Model file for the job. Use its own axes, mm. Face numbers are marked on the shaded views. A direction names the side the tool comes from. Give positions to 0.01 mm unless a question says otherwise; leave off trailing zeros. Loops run counter-clockwise (first coordinate to the right, second up) from the corner with the lowest first, then second, coordinate; pieces in that order, holes last. Notation, with made-up numbers: (-12.5, 66.25) - (26.5, 66.25) arc R25 ccw to (26.5, 90.25) - close; hole circle Ø8 at (19, 36). An arc over 180 degrees is marked (long way). Use a Markdown table: item, result.
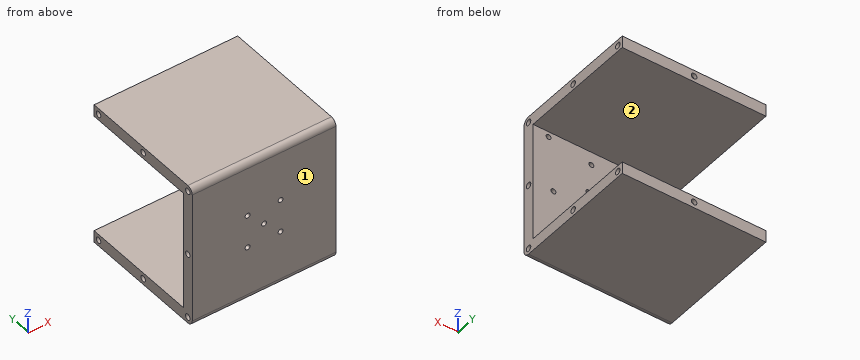
Autodesk Inventor part; units mm, degrees
ref_plane "YZ Plane" through (0, 0, 0) normal (1, 0, 0) x (0, 1, 0)
ref_plane "XZ Plane" through (0, 0, 0) normal (0, 1, 0) x (-1, 0, 0)
ref_plane "XY Plane" through (0, 0, 0) normal (0, 0, 1) x (1, 0, 0)
sketch "Sketch1" plane through (0, 0, 0) normal (0, 1, 0) x (-1, 0, 0)
  point P0 (0, 0)
sketch "Sketch2" plane through (0, 0, 0) normal (0, 1, 0) x (-1, 0, 0)
  line L0 (-76.2, 76.2) -> (76.2, 76.2)
  line L1 (76.2, 76.2) -> (76.2, -76.2)
  line L2 (76.2, -76.2) -> (-76.2, -76.2)
  line L3 (-76.2, -76.2) -> (-76.2, 76.2)
  line L4 (-76.2, 76.2) -> (76.2, -76.2) construction
  line L5 (76.2, 76.2) -> (-76.2, -76.2) construction
  point P0 (0, 0)
  dimension "d0" = 152.4
  dimension "d1" = 152.4
extrude "Extrusion1" add sketch "Sketch2" along normal blind 12.7
sketch "Sketch3" plane through (0, 12.7, 0) normal (0, 1, 0) x (1, 0, 0)
  line L0 (76.2, 76.2) -> (-76.2, 76.2)
  line L1 (76.2, -76.2) -> (76.2, 76.2)
  line L2 (-76.2, 76.2) -> (76.2, 76.2)
  line L3 (76.2, 76.2) -> (76.2, 63.5)
  line L4 (76.2, 63.5) -> (-76.2, 63.5)
  line L5 (-76.2, 63.5) -> (-76.2, 76.2)
  line L6 (-76.2, -76.2) -> (76.2, -76.2)
  line L7 (76.2, -76.2) -> (76.2, -63.5)
  line L8 (76.2, -63.5) -> (-76.2, -63.5)
  line L9 (-76.2, -63.5) -> (-76.2, -76.2)
  point P0 (0, 0)
  point P1 (76.2, -76.2)
  dimension "d4" = 12.7
  dimension "d5" = 12.7
  dimension "d15" = 152.4
extrude "Extrusion2" add sketch "Sketch3" along normal blind 127
fillet "Fillet1" radius 6.35 2 edges at (0, 0, 76.2) (0, 0, -76.2)
sketch "Sketch4" plane through (76.2, 12.7, -63.5) normal (1, 0, 0) x (0, 0, -1)
  circle A0 centre (-133.35, 120.65) radius 3.175
  circle A1 centre (-133.35, -6.35) radius 3.175
  circle A2 centre (-133.35, 57.15) radius 3.175
  circle A3 centre (6.35, 120.65) radius 3.175
  circle A4 centre (6.35, -6.35) radius 3.175
  circle A5 centre (6.35, 57.15) radius 3.175
  circle A6 centre (-63.5, -6.35) radius 3.175
  point P0 (-63.5, -12.7)
  dimension "d9" = 127
extrude "Extrusion3" cut sketch "Sketch4" against normal blind 12.7
sketch "Sketch5" plane through (-76.2, 12.7, 63.5) normal (-1, 0, 0) x (0, 0, 1)
  circle A0 centre (-133.35, 120.65) radius 3.175
  circle A1 centre (-133.35, 120.65) radius 3.175
  circle A2 centre (-133.35, 57.15) radius 3.175
  circle A3 centre (-133.35, 57.15) radius 3.175
  circle A4 centre (-133.35, -6.35) radius 3.175
  circle A5 centre (-133.35, -6.35) radius 3.175
  circle A6 centre (-63.5, -6.35) radius 3.175
  circle A7 centre (-63.5, -6.35) radius 3.175
  circle A8 centre (6.35, -6.35) radius 3.175
  circle A9 centre (6.35, -6.35) radius 3.175
  circle A10 centre (6.35, 57.15) radius 3.175
  circle A11 centre (6.35, 57.15) radius 3.175
  circle A12 centre (6.35, 120.65) radius 3.175
  circle A13 centre (6.35, 120.65) radius 3.175
  line L0 (6.35, -12.7) -> (-133.35, -12.7)
  point P0 (-63.5, -12.7)
  dimension "d20" = 69.85
sketch "Sketch6" plane through (0, 139.7, 0) normal (0, 1, 0) x (1, 0, 0)
  line L0 (76.2, 69.85) -> (-76.2, 69.85)
  circle A0 centre (0, 69.85) radius 3
  line L1 (-76.2, -69.85) -> (76.2, -69.85)
  circle A1 centre (0, -69.85) radius 3
  point P0 (0, 0)
  dimension "d16" = 6
  dimension "d17" = 6
extrude "Extrusion5" cut sketch "Sketch6" against normal blind 4
extrude "Extrusion6" cut sketch "Sketch5" against normal blind 12.7
sketch "Sketch7" plane through (0, 12.7, 0) normal (0, 1, 0) x (1, 0, 0)
  line L0 (76.2, 0) -> (63.5, 0)
  line L1 (63.5, 3.175) -> (63.5, -3.175)
  line L2 (63.5, 0) -> (57.15, 0)
  circle A0 centre (54.5465, 0) radius 2.6035
  line L3 (51.943, 0) -> (-35.687, 0)
  line L4 (-35.687, 0) -> (-35.687, 35.56)
  line L5 (-35.687, 35.56) -> (-35.687, -35.56)
  circle A1 centre (-35.687, 38.1635) radius 2.6035
  circle A2 centre (-35.687, -38.1635) radius 2.6035
  point P0 (0, 0)
  dimension "d28" = 5.207
  dimension "d29" = 5.207
  dimension "d23" = 6.35
  dimension "d24" = 5.207
  dimension "d25" = 87.63
  dimension "d26" = 35.56
  dimension "d27" = 71.12
extrude "Extrusion7" cut sketch "Sketch7" against normal blind 3.9878
sketch "Sketch8" plane through (0, 12.7, 0) normal (0, 1, 0) x (1, 0, 0)
  circle A0 centre (54.5465, 0) radius 2.6035
  line L0 (51.943, 0) -> (-76.2, 0)
  point P0 (0, 0)
sketch "Sketch9" plane through (0, 12.7, 0) normal (0, 1, 0) x (1, 0, 0)
  point P0 (0, 0)
sketch "Sketch10" plane through (0, 12.7, 0) normal (0, 1, 0) x (1, 0, 0)
  line L0 (57.15, -63.5) -> (57.15, -52.07)
  line L1 (57.15, -57.785) -> (-19.177, -57.785)
  line L2 (-76.2, -63.5) -> (76.2, -63.5)
  line L3 (13.97, -63.5) -> (13.97, -52.07)
  line L4 (11.1125, -52.07) -> (17.4625, -52.07)
  circle A0 centre (14.2875, -49.4665) radius 2.6035
  circle A1 centre (59.7535, -57.785) radius 2.6035
  line L5 (-19.177, -61.9125) -> (-19.177, -53.133)
  circle A2 centre (-21.7805, -57.785) radius 2.6035
  point P0 (0, 0)
  dimension "d32" = 11.43
  dimension "d33" = 76.327
  dimension "d36" = 5.207
  dimension "d37" = 5.207
  dimension "d38" = 5.207
extrude "Extrusion8" cut sketch "Sketch10" against normal blind 3.9878 contours A2 | A0 | A1
sketch "Sketch11" plane through (0, 0, 0) normal (0, -1, 0) x (1, 0, 0)
  line L0 (17.526, -17.526) -> (-17.526, -17.526)
  line L1 (-17.526, -17.526) -> (-17.526, 17.526)
  line L2 (-17.526, 17.526) -> (17.526, 17.526)
  line L3 (17.526, 17.526) -> (17.526, -17.526)
  line L4 (17.526, -17.526) -> (-17.526, 17.526) construction
  line L5 (-17.526, -17.526) -> (17.526, 17.526) construction
  circle A0 centre (-50.8, 55.5625) radius 2.6035
  circle A1 centre (-17.526, 17.526) radius 2.6035
  circle A2 centre (-17.526, -17.526) radius 2.6035
  circle A3 centre (17.526, -17.526) radius 2.6035
  circle A4 centre (17.526, 17.526) radius 2.6035
  point P0 (0, 0)
  dimension "d39" = 35.052
  dimension "d40" = 35.052
  dimension "d41" = 5.207
  dimension "d42" = 5.207
  dimension "d43" = 5.207
  dimension "d44" = 5.207
  dimension "d45" = 5.207
extrude "Extrusion9" cut sketch "Sketch11" along normal blind 25.4 and the other way blind 25.4 contours A2 L1 L0 | L0 L1 A2 | A3 L3 L0 | L0 L3 A3 | A1 L2 L1 | L1 L2 A1 | A4 L2 L3 | L3 L2 A4
sketch "Sketch13" plane through (0, 12.7, 0) normal (0, 1, 0) x (1, 0, 0)
  circle A0 centre (0, 0) radius 2.6035
  dimension "d54" = 5.207
extrude "Extrusion11" cut sketch "Sketch13" against normal blind 25.4
properties part number "Fuselage_Body_Piece"
(1) Slice it at C-C, the plane y = 50. Write the cut outline in (x, z), plus the area to 3 significant figures.
Computed:
| item | result |
|---|---|
| outline | (-76.2, -76.2) - (76.2, -76.2) - (76.2, -63.5) - (-76.2, -63.5) - close; (-76.2, 63.5) - (76.2, 63.5) - (76.2, 76.2) - (-76.2, 76.2) - close |
| area | 3,870 mm² |
(2) Pin check, flat tips, straight feed: P1, Ø5, axis at x = 0, z = -70, coming from the +Y side; P2, Ø6, axis at x = -21.78, z = 57.78, coming from the -Y side; P3, Ø5.5, axis at x = 14.5, z = 49.5, coming from the +Y side; P4, Ø1.9, axis at y = 134.5, z = -71.5, coming from the -X side. Stop position of each tip, or through.
Computed:
| item | result |
|---|---|
| P1 | y = 135.7 |
| P2 | y = 0 |
| P3 | y = 12.7 |
| P4 | x = -63.5 |
(3) Slice it at D-D, the plane x = 44. Write the cut outline in (y, z), plus the area to 3 significant figures.
Computed:
| item | result |
|---|---|
| outline | (0, -69.85) arc R6.35 ccw to (6.35, -76.2) - (139.7, -76.2) - (139.7, -63.5) - (12.7, -63.5) - (12.7, 63.5) - (139.7, 63.5) - (139.7, 76.2) - (6.35, 76.2) arc R6.35 ccw to (0, 69.85) - close |
| area | 5,140 mm² |
(4) 3-axis set-ups, long thin cutter, end or side, ignore diameter. For the marked faces 1 and 2: which of +Z, -Z, +X, -X, +Y, -Y reach the whole face in a straight line?
Computed:
| item | result |
|---|---|
| face 1 | +Z, -Z, +X, -X, -Y |
| face 2 | +X, -X, +Y |
(5) Slice it at A-A, the plane y = 69.85. Write the cut outline in (x, z) (3 decimals).
Computed:
| item | result |
|---|---|
| outline | (-76.2, -76.2) - (76.2, -76.2) - (76.2, -73.025) - (63.5, -73.025) - (63.5, -66.675) - (76.2, -66.675) - (76.2, -63.5) - (-76.2, -63.5) - (-76.2, -66.675) - (-63.5, -66.675) - (-63.5, -73.025) - (-76.2, -73.025) - close; (-76.2, 63.5) - (76.2, 63.5) - (76.2, 66.675) - (63.5, 66.675) - (63.5, 73.025) - (76.2, 73.025) - (76.2, 76.2) - (-76.2, 76.2) - (-76.2, 73.025) - (-63.5, 73.025) - (-63.5, 66.675) - (-76.2, 66.675) - close |
(6) Slice it at B-B, the plane x = 0. Write the cut outline in (y, z), plus the area to 3 significant figures.
Computed:
| item | result |
|---|---|
| outline | (0, -69.85) arc R6.35 ccw to (6.35, -76.2) - (139.7, -76.2) - (139.7, -72.85) - (135.7, -72.85) - (135.7, -66.85) - (139.7, -66.85) - (139.7, -63.5) - (12.7, -63.5) - (12.7, -2.6) - (0, -2.6) - close; (0, 2.6) - (12.7, 2.6) - (12.7, 63.5) - (139.7, 63.5) - (139.7, 66.85) - (135.7, 66.85) - (135.7, 72.85) - (139.7, 72.85) - (139.7, 76.2) - (6.35, 76.2) arc R6.35 ccw to (0, 69.85) - close |
| area | 5,030 mm² |
(7) Drill centre lines: probe 1 along Z at (x, y) = (-68, 133.35) (3 decimals); probe 2 along Y at (x, z) = (69.5, -69.85) (3 decimals); probe 3 along Z at (x, y) = (-52.5, 91). Where is each one in solid material? Low to high. Write a range as [from, to].
Computed:
| item | result |
|---|---|
| probe 1 | [-76.2, -73.025], [-66.675, -63.5], [63.5, 66.675], [73.025, 76.2] |
| probe 2 | [0, 3.175], [9.525, 66.675], [73.025, 130.175], [136.525, 139.7] |
| probe 3 | [-76.2, -63.5], [63.5, 76.2] |
